Source: CAD feature listing. Evaluate the final solid. Frame: model axes, mm. A direction names the side the tool comes from. Round coordinates to 2 decimals unless told otherwise and drop trailing zeros. Use a Markdown table: item, result.
Autodesk Inventor part; units mm, degrees
ref_plane "YZ Plane" through (0, 0, 0) normal (1, 0, 0) x (0, 1, 0)
ref_plane "XZ Plane" through (0, 0, 0) normal (0, 1, 0) x (-1, 0, 0)
ref_plane "XY Plane" through (0, 0, 0) normal (0, 0, 1) x (1, 0, 0)
sketch "Sketch1" plane through (0, 0, 0) normal (0, 0, 1) x (1, 0, 0)
  line L0 (0, 0) -> (127, 0)
  line L1 (127, 0) -> (127, 50.8)
  line L2 (127, 50.8) -> (0, 50.8)
  line L3 (0, 50.8) -> (0, 0)
  dimension "d0" = 127
  dimension "d1" = 50.8
extrude "Extrusion1" add sketch "Sketch1" along normal blind 12.7
sketch "Sketch2" plane through (0, 0, 12.7) normal (0, 0, 1) x (1, 0, 0)
  line L0 (127, 0) -> (0, 0)
  line L1 (0, 50.8) -> (127, 50.8)
  line L2 (63.5, 50.8) -> (66.5874, 50.8)
  line L3 (66.5874, 50.8) -> (66.5874, 0)
  line L4 (66.5874, 0) -> (63.5, 0)
  line L5 (63.5, 0) -> (63.5, 50.8)
extrude "Extrusion2" cut sketch "Sketch2" against normal blind 2.54
sketch "Sketch3" plane through (0, 0, 0) normal (0, 0, -1) x (-1, 0, 0)
  line L0 (0, 0) -> (-127, 0)
  line L1 (-127, 50.8) -> (0, 50.8)
  line L2 (-63.5, 50.8) -> (-66.7421, 50.8)
  line L3 (-66.7421, 50.8) -> (-66.7421, 0)
  line L4 (-66.7421, 0) -> (-63.5, 0)
  line L5 (-63.5, 0) -> (-63.5, 50.8)
extrude "Extrusion3" cut sketch "Sketch3" against normal blind 2.54
properties part number "Magnet"
Q1. Reachability of faces 1 (the flat face through (66.587, 26, 11)), 2 (the flat face through (66.742, 26, 1)), 3 (the flat face through (96, 26, 0)) from +Z, -Z, +X, -X, +Y, -Y: full face, straight path, thin tool, end or side. Return the list, or none.
Results are:
| item | result |
|---|---|
| face 1 | +Z, +Y, -Y |
| face 2 | -Z, +Y, -Y |
| face 3 | -Z, +X, -X, +Y, -Y |
Q2. Mould query, pull axis X, two halves, no side actions, for faces 4 (the flat face through (63.5, 25, 1)), 5 (the flat face through (63, 0, 6)), 6 (the flat face through (0, 26, 6)). Classes: +X half, -X half, draft (parallel to the pull), parting line (faces both ways), or undercut.
Results are:
| item | result |
|---|---|
| face 4 | undercut |
| face 5 | draft |
| face 6 | -X half |
Q3. First-contact query: pin 1 Ø1.5 at (x, y) = (65.5, 25.5) entering from +Z; pin 2 Ø1 at (x, y) = (65, 32) entering from -Z. Flat tips, straight axial feed; report the tip coordinate or a pass-through.
Results are:
| item | result |
|---|---|
| pin 1 | z = 10.16 |
| pin 2 | z = 2.54 |
Q4. Line query: L1, parallel to X at y = 32, z = 12.25; L2, parallel to X at y = 6.5, z = 2.5; L3, parallel to Z at x = 65, y = 43.5. Output: solid intervals per line, ascending.
Results are:
| item | result |
|---|---|
| L1 | 0 to 63.5, 66.59 to 127 |
| L2 | 0 to 63.5, 66.74 to 127 |
| L3 | 2.54 to 10.16 |
